For this review, take the finished solid that the model builds, in its own axes (mm). A direction names the side the tool comes from. Give positions to 0.01 mm unless a question says otherwise; leave off trailing zeros. Loops run counter-clockwise (first coordinate to the right, second up) from the corner with the lowest first, then second, coordinate; pieces in that order, holes last. Notation, with made-up numbers: (64.5, 4.5) - (98.5, 4.5) arc R13 cw to (98.5, 19.5) - close; hole circle Ø5 at (27, -15). An arc over 180 degrees is marked (long way). Put each result on its own line as item: value. Start each with the question number.
from build123d import *

# Parameters (mm, degrees)
BOSS_EXTRUDE1_DEPTH = 3.175
SKETCH2_W           = 3.175
SKETCH2_H           = 42.3
BOSS_EXTRUDE2_DEPTH = 14.29
SKETCH3_R           = 1.6
BOSS_EXTRUDE3_DEPTH = 3.175


with BuildPart() as part:
    # Sketch1 → Boss-Extrude1 (new body)
    with BuildSketch(Plane(origin=(0, 0, 0), x_dir=(1, 0, 0), z_dir=(0, 1, 0))):
        with BuildLine():
            Line((0, 0), (20, 0))
            Line((20, 0), (20, -42.3))
            Line((20, -42.3), (0, -42.3))
            ThreePointArc((0, -42.3), (8.723780881, -21.15), (0, 0))
        make_face()
    boss_extrude1 = extrude(amount=BOSS_EXTRUDE1_DEPTH)

    # Sketch2 → Boss-Extrude2 (add)
    with BuildSketch(Plane(origin=(0, 3.175, 0), x_dir=(1, 0, 0), z_dir=(0, 1, 0))):
        with Locations((18.4125, -21.15)):
            Rectangle(SKETCH2_W, SKETCH2_H)
    extrude(amount=BOSS_EXTRUDE2_DEPTH)

    # Mirror1: Boss-Extrude1 across plane
    add(boss_extrude1.mirror(Plane.ZX.offset(10.32)))

    # Sketch3 → Boss-Extrude3 (add)
    with BuildSketch(Plane(origin=(0, 0, 0), x_dir=(-1, 0, 0), z_dir=(0, 0, -1))):
        with BuildLine():
            Line((-20, 0), (0, 0))
            Line((0, 0), (0, 6.32))
            Line((0, 6.32), (-6, 6.32))
            ThreePointArc((-6, 6.32), (-10, 10.32), (-6, 14.32))
            Line((-6, 14.32), (0, 14.32))
            Line((0, 14.32), (0, 20.64))
            Line((0, 20.64), (-20, 20.64))
            Line((-20, 20.64), (-20, 0))
        make_face()
        with Locations((-13.825, 6.32)):
            Circle(SKETCH3_R, mode=Mode.SUBTRACT)
        with Locations((-13.825, 14.32)):
            Circle(SKETCH3_R, mode=Mode.SUBTRACT)
    boss_extrude3 = extrude(amount=BOSS_EXTRUDE3_DEPTH)

    # Mirror2: Boss-Extrude3 across plane
    add(boss_extrude3.mirror(Plane.XY.offset(21.15)))


solid = part.part
1) Take a section at D-D on z = 40.5. State the section outline as (x, y) points (3 decimals), and give its area (3 significant figures).
2) Wall thickness on probe 1 along Y at (x, z) = (5.5, 41.5) (3 decimals); probe 2 along Z at (x, y) = (6.5, 17.25) (3 decimals); probe 3 along X at (y, z) = (13.75, 35) (3 decimals): over which ranges is each line inside the solid? List them lowest first.
3) Take a section at A-A on x = 11.5. State the section outline as (y, z) points (3 decimals), and give its area (3 significant figures).
4) Machinability: for faces 1 (the flat face through (3, 14.32, -2)), 2 (the flat face through (10, 17.465, 21)), 3 (the flat face through (0, 3, -2)), which of the approach directions +Z, -Z, +X, -X, +Y, -Y give a long, thin tool a straight path to every point of the face, cutting with its end or side? Answer none if there is none.
5) Take a section at C-C on y = 10.32. State the section outline as (x, z) points (3 decimals).
6) Take a section at B-B on y = 7. State the section outline as (x, z) points (3 decimals), and give its area (3 significant figures).
7) Mouldability with a two-part tool opening along Z and no side actions: class faces 4 (the flat face through (12, 10, 45.475)), 5 (the flat face through (3, 6.32, 44)), 6 (the cylindrical face through (8.72, 19.07, 21.48)) as released by +Z, released by -Z, zero draft, split by the parting line, or undercut.
8) Insertion check: P1, Ø7, axis at y = 10.5, z = 26.5, coming from the -X side (3 decimals). The pin has a flat end and moves straight along its axis. Give the tip position at first contact, or say it passes through.
Answers follow:
1. outline: (1.649, 0) - (20, 0) - (20, 20.64) - (1.649, 20.64) - (1.649, 17.465) - (16.825, 17.465) - (16.825, 3.175) - (1.649, 3.175) - close
1. area: 162 mm2
2. probe 1: 0 to 3.175, 17.465 to 20.64
2. probe 2: -3.175 to 0, 42.3 to 45.475
2. probe 3: 16.825 to 20
3. outline: (0, -3.175) - (20.64, -3.175) - (20.64, 45.475) - (0, 45.475) - close; hole (3.175, 0) - (17.465, 0) - (17.465, 42.3) - (3.175, 42.3) - close
3. area: 400 mm2
4. face 1: +Z, -Z, -X
4. face 2: -X
4. face 3: +Z, -Z, -X, +Y, -Y
5. outline: (10, -3.175) - (20, -3.175) - (20, 45.475) - (10, 45.475) - (10, 42.3) - (16.825, 42.3) - (16.825, 0) - (10, 0) - close
6. outline: (8.231, -3.175) - (12.377, -3.175) - (12.377, 0) - (8.231, 0) - close; (8.231, 42.3) - (12.377, 42.3) - (12.377, 45.475) - (8.231, 45.475) - close; (15.273, -3.175) - (20, -3.175) - (20, 45.475) - (15.273, 45.475) - (15.273, 42.3) - (16.825, 42.3) - (16.825, 0) - (15.273, 0) - close
6. area: 191 mm2
7. face 4: released by +Z
7. face 5: zero draft
7. face 6: undercut
8. P1: x = 16.825
